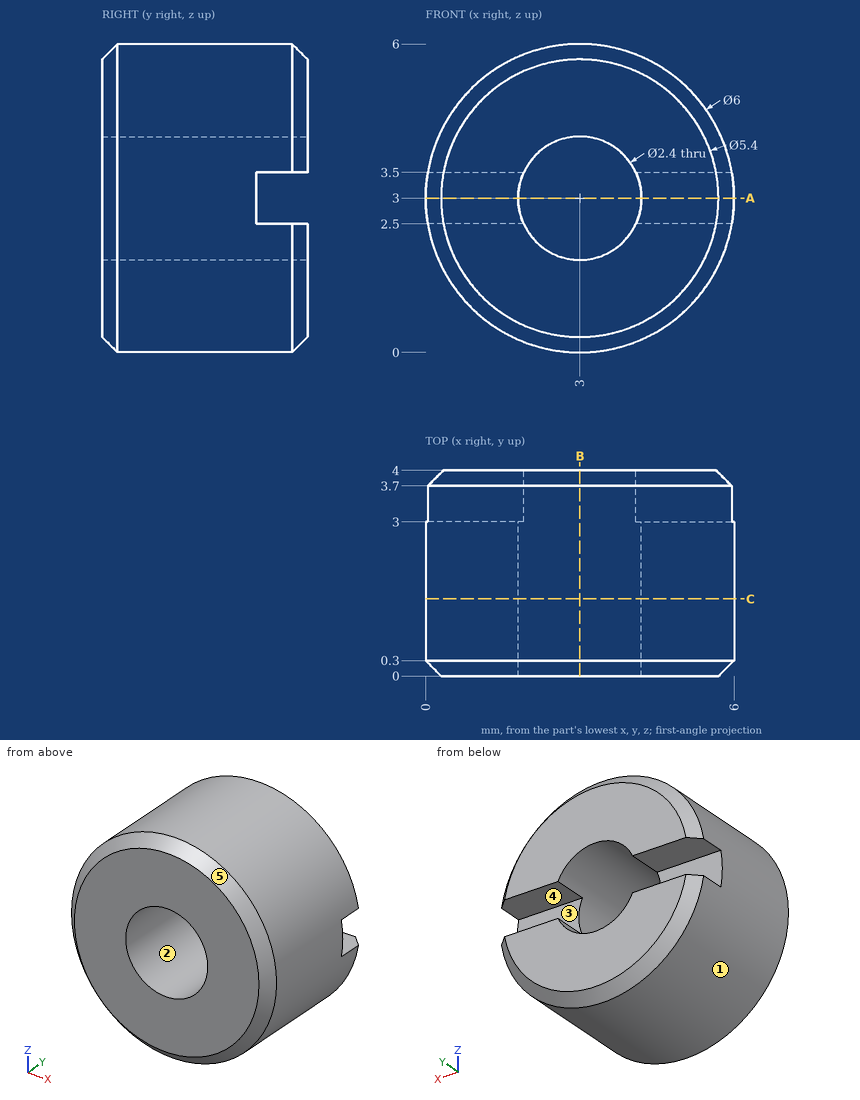
Study the drawing (mm; zero at the part's minimum x, y, z) and answer. A direction names the side the tool comes from. Coordinates: 2 decimals unless noted, no trailing zeros. Write each loop counter-clockwise with the first axis right and the second up, starting at its lowest first coordinate (ties: lowest second). Pieces come first, ordered by that corner, then holes. Notation, with made-up numbers: M 30.25,34.5 L 38.25,34.5 A23 ccw 38.25,62.5 Z; hole C -1.75,-29 d8. An arc over 180 degrees is marked long. Write each question's results on one line, items separated by ' | '.
Item 1: The part is cut by section C-C on y = 1.5. Determine the outline of the cut face in (x, z), and give its area (3 significant figures).
Answer below:
outline: C 3,3 d6; hole C 3,3 d2.4 | area: 23.8 mm2
Item 2: Given P1, Ø0.5, axis at x = 5, z = 3, coming from the +Y side; P2, Ø1, axis at y = 2.5, z = 1, coming from the -X side; P3, Ø0.8, axis at x = 1, y = 3.5, coming from the +Z side; P4, Ø1.9, axis at x = 3, z = 3, coming from the -Y side, each flat-ended and moving along its own axis, determine where each tip first touches the part or whether it passes through.
Answer below:
P1: y = 3 | P2: x = 0.4 | P3: z = 5.54 | P4: through
Item 3: Consider probe 1 along Z at (x, y) = (3, 2.75); probe 2 along Y at (x, z) = (0.75, 2.95). Determine where each line is inside the solid, lowest interval first. Write a range as [from, to].
Answer below:
probe 1: [0, 1.8], [4.2, 6] | probe 2: [0, 3]
Item 4: For a pull along X with two mould halves and no side action, classify the marked faces 1, 2 and 3 as released by +X, released by -X, zero draft, split by the parting line, or undercut.
Answer below:
face 1: split by the parting line | face 2: undercut | face 3: zero draft
Item 5: Which of the six approach directions +Z, -Z, +X, -X, +Y, -Y give full straight-line access (tool end or side, diameter ignored) to the marked faces 4 and 5?
Answer below:
face 4: +X, -X, +Y | face 5: -Y
Item 6: The part is cut by section B-B on x = 3. Determine the outline of the cut face in (y, z).
Answer below:
outline: M 0,0.3 L 0.3,0 L 3.7,0 L 4,0.3 L 4,1.8 L 0,1.8 Z; M 0,4.2 L 4,4.2 L 4,5.7 L 3.7,6 L 0.3,6 L 0,5.7 Z
Item 7: The part is cut by section A-A on z = 3. Determine the outline of the cut face in (x, y).
Answer below:
outline: M 0,0.3 L 0.3,0 L 1.8,0 L 1.8,3 L 0,3 Z; M 4.2,0 L 5.7,0 L 6,0.3 L 6,3 L 4.2,3 Z
